Here's the drawing with two shaded views (mm, measured from the low corner). I have some questions. A direction names the side the tool comes from. Give positions to 0.01 mm unless a question says otherwise; leave off trailing zeros. Loops run counter-clockwise (first coordinate to the right, second up) from the corner with the lowest first, then second, coordinate; pieces in that order, holes last. Notation, with made-up numbers: M -35.5,77.5 L -10.5,77.5 A3 ccw -10.5,82.5 Z; hole C 86.5,18 d10. An arc over 180 degrees is marked long. Use a Markdown table: item, result. Add a question column.
1) If I drill on line 1 along Z through (x, y) = (7.25, 13.75); line 2 along Z through (x, y) = (8.75, 19.5); line 3 along Z through (x, y) = (4.25, 18.75) (1 decimal), over which ranges is the centre line in solid material (lowest first)? Write a range as [from, to].
2) Which directions (+Z, -Z, +X, -X, +Y, -Y) give clear straight access to the entire face, cutting with the end or side of a thin tool? Please do the marked faces 4, 5 and 6.
3) We'd pull the mould along Y, two halves only. Please class the marked faces 1, 2 and 3: +Y half, -Y half, draft (parallel to the pull), parting line (faces both ways), or undercut.
4) Suppose I cut it at C-C on z = 7.75. List the corners of the cut face in (x, y) for me.
5) Suppose I cut it at D-D on y = 20.25. List the corners of the cut face in (x, z) for me.
6) Suppose I cut it at A-A on y = 9. List the corners of the cut face in (x, z) for me.
7) Will this pin go through, and if not, where does the flat tip stop? pin 1 Ø4 at (y, z) = (9.5, 6) entering from -X.
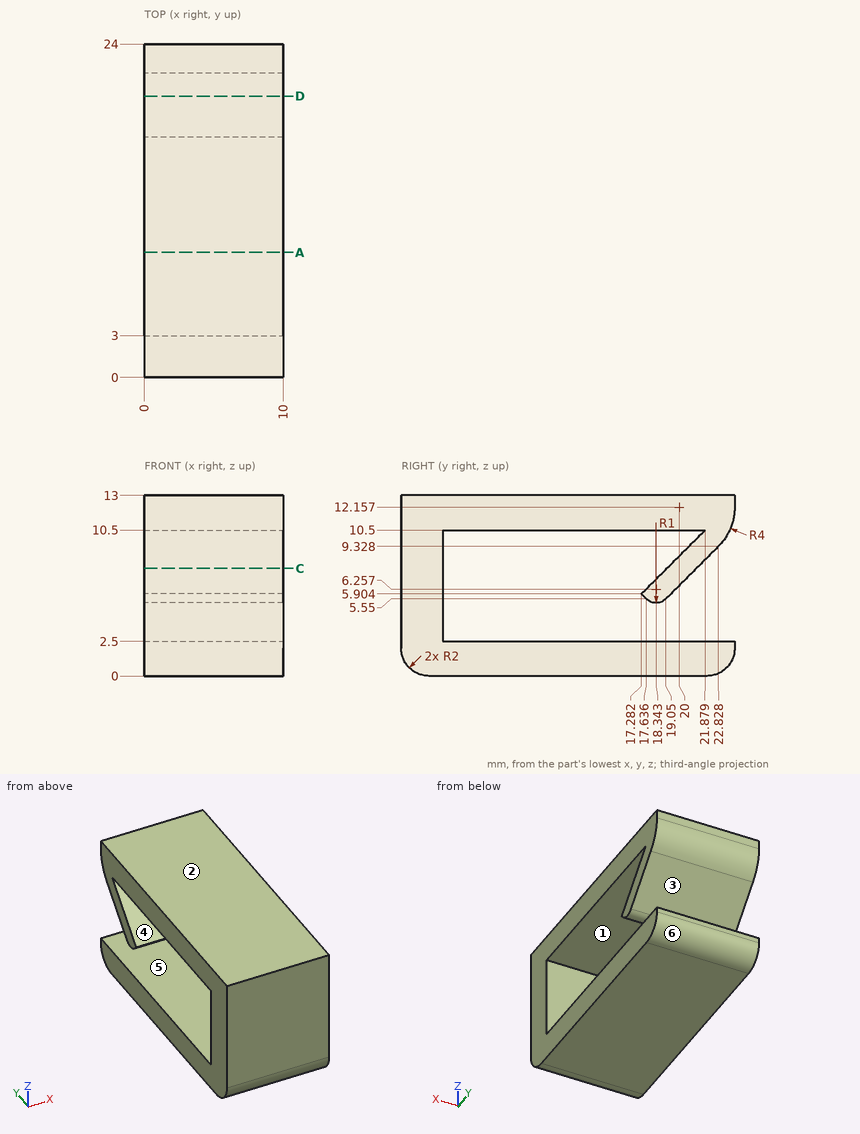
Answer block:
| question | item | result |
|---|---|---|
| 1 | line 1 | z = [0, 2.5], [10.5, 13] |
| 1 | line 2 | z = [0, 2.5], [6, 8.12], [10.5, 13] |
| 1 | line 3 | z = [0, 2.5], [5.3, 7.4], [10.5, 13] |
| 2 | face 4 | +X, -X |
| 2 | face 5 | +X, -X, +Y |
| 2 | face 6 | -Z, +X, -X, +Y |
| 3 | face 1 | undercut |
| 3 | face 2 | draft |
| 3 | face 3 | +Y half |
| 4 | outline | M 0,0 L 10,0 L 10,3 L 0,3 Z; M 0,19.13 L 10,19.13 L 10,21.25 L 0,21.25 Z |
| 5 | outline | M 0,0 L 10,0 L 10,2.5 L 0,2.5 Z; M 0,6.75 L 10,6.75 L 10,8.87 L 0,8.87 Z; M 0,10.5 L 10,10.5 L 10,13 L 0,13 Z |
| 6 | outline | M 0,0 L 10,0 L 10,2.5 L 0,2.5 Z; M 0,10.5 L 10,10.5 L 10,13 L 0,13 Z |
| 7 | pin 1 | passes through |
